Source: CAD feature listing. Evaluate the final solid. Frame: model axes, mm. Face numbers are marked on the shaded views. Coordinates: 2 decimals unless noted, no trailing zeros. Order: outer loops, then holes, each group sorted by start corner. A loop starts at its lowest first (then second) coordinate and runs counter-clockwise, first axis right, second up. Notation, with made-up numbers: (-1.75, 13.25) -> (11.25, 13.25) arc R20 cw to (11.25, 26.25) -> close; hole circle Ø8 at (-32, 20.25). An arc over 180 degrees is marked (long way). Write each question's results on one line, items separated by ' | '. Start each with the question number.
from build123d import *

# Parameters (mm, degrees)
SKETCH1_R          = 200
EXTRUDE1_DEPTH     = 20
SKETCH2_R          = 17.5
CUT_EXTRUDE1_DEPTH = 10


with BuildPart() as part:
    # Sketch1 → Extrude1 (new body)
    with BuildSketch(Plane(origin=(0, 0, 0), x_dir=(1, 0, 0), z_dir=(0, 1, 0))):
        with Locations(Location((0, 0, 0), (0, 0, 270))):
            Circle(SKETCH1_R)
    extrude(amount=-EXTRUDE1_DEPTH)

    # Sketch2 → Cut-Extrude1 (cut)
    with BuildSketch(Plane(origin=(0, 0, 0), x_dir=(1, 0, 0), z_dir=(0, 1, 0))):
        with Locations(Location((0, 170, 0), (0, 0, 270))):
            Circle(SKETCH2_R)
        with Locations(Location((43.999237667, 164.207390469, 0), (0, 0, 270))):
            Circle(SKETCH2_R)
        with Locations(Location((147.224318643, -85, 0), (0, 0, 270))):
            Circle(SKETCH2_R)
        with Locations(Location((120.208152802, -120.208152802, 0), (0, 0, 270))):
            Circle(SKETCH2_R)
        with Locations(Location((-147.224318643, -85, 0), (0, 0, 270))):
            Circle(SKETCH2_R)
        with Locations(Location((-164.207390469, -43.999237667, 0), (0, 0, 270))):
            Circle(SKETCH2_R)
    extrude(amount=-CUT_EXTRUDE1_DEPTH, mode=Mode.SUBTRACT)


solid = part.part
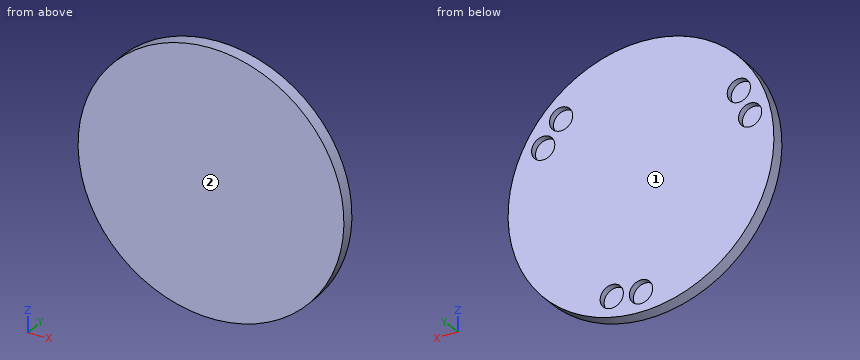
(1) Section C-C on y = -16. Return the cut outline in (x, z).
(2) Section B-B on z = -170. Return the cut outline in (x, y), then the cut area to 3 significant figures.
(3) Line query: L1, parallel to X at y = -5.75, z = -175; L2, parallel to X at y = -3.5, z = -170; L3, parallel to Z at x = 147, y = -3.75. Output: solid intervals per line, ascending.
(4) Section A-A on x = 0. Return the cut outline in (y, z).
(5) Draft query along Y for the marked faces 1 and 2. Return one class per face: released by +Y, released by -Y, zero draft, split by the parting line, or undercut.
(6) Section D-D on z = 43. Return the cut outline in (x, y), then the cut area to 3 significant figures.
(7) First-contact query: P1, Ø4, axis at x = 122.5, y = -4, coming from the +Z side; P2, Ø1, axis at y = -17.5, z = -78, coming from the +X side; P3, Ø4, axis at x = -59.5, y = -9, coming from the -Z side; P4, Ø1.5, axis at x = -107, z = -76, coming from the +Y side. Flat tips, straight axial feed; report the tip coordinate or a pass-through.
Results list:
1) outline: circle Ø400 at (0, 0)
2) outline: (-105.36, -20) -> (105.36, -20) -> (105.36, 0) -> (60.51, 0) -> (60.51, -10) -> (27.49, -10) -> (27.49, 0) -> (17.5, 0) -> (17.5, -10) -> (-17.5, -10) -> (-17.5, 0) -> (-105.36, 0) -> close | area: 3,530 mm²
3) L1: x = -96.82 to -16.77, 16.77 to 30.22, 57.77 to 96.82 | L2: x = -105.36 to -17.5, 17.5 to 27.49, 60.51 to 105.36 | L3: z = -135.61 to 67.5, 102.5 to 135.61
4) outline: (-20, -200) -> (0, -200) -> (0, -187.5) -> (-10, -187.5) -> (-10, -152.5) -> (0, -152.5) -> (0, 200) -> (-20, 200) -> close
5) face 1: released by +Y | face 2: released by -Y
6) outline: (-195.32, -20) -> (195.32, -20) -> (195.32, 0) -> (-146.74, 0) -> (-146.74, -10) -> (-181.68, -10) -> (-181.68, 0) -> (-195.32, 0) -> close | area: 7,460 mm²
7) P1: stops at z = 159.62 | P2: stops at x = 184.37 | P3: stops at z = -191.56 | P4: stops at y = 0
